Input: part model. Units: mm. Frame: model coordinates. A direction names the side the tool comes from. Coordinates: 2 decimals unless noted, no trailing zeros. Write each loop counter-clockwise with the first axis right and the second up, starting at its lowest first coordinate (ties: lowest second). Pieces come first, ordered by that corner, then holes. Notation, with made-up numbers: M 62,88.25 L 83,88.25 A36 ccw 83,125.25 Z; hole C 10,0.25 d8. An arc over 180 degrees is marked long. Use one line per item in the form item = value.
from build123d import *

# Parameters (mm, degrees)
EXTRUDE003_DEPTH = 5
EXTRUDE002_DEPTH = 5


with BuildPart() as extrude003:
    # Sketch010 (on Face2 of Cut) → Extrude003 (new body)
    with BuildSketch(Plane(origin=(0, 0, 0), x_dir=(1, 0, 0), z_dir=(0, 0, -1))):
        with BuildLine():
            Line((-28.464466, 33.464466), (28.464466, 33.464466))
            ThreePointArc((33.464466, 28.464466), (32, 32), (28.464466, 33.464466))
            Line((33.464466, 28.464466), (33.464466, -28.464466))
            ThreePointArc((28.464466, -33.464466), (32, -32), (33.464466, -28.464466))
            Line((28.464466, -33.464466), (-28.464466, -33.464466))
            ThreePointArc((-33.464466, -28.464466), (-32, -32), (-28.464466, -33.464466))
            Line((-33.464466, -28.464466), (-33.464466, 28.464466))
            ThreePointArc((-28.464466, 33.464466), (-32, 32), (-33.464466, 28.464466))
        make_face()
    extrude(amount=EXTRUDE003_DEPTH)


with BuildPart() as obj1:
    # Sketch009 (on Face2 of Cut) → Extrude002 (new body)
    with BuildSketch(Plane(origin=(0, 0, 0), x_dir=(1, 0, 0), z_dir=(0, 0, -1))):
        with BuildLine():
            ThreePointArc((-31.464466, 36.464466), (-35, 35), (-36.464466, 31.464466))
            Line((-36.464466, -31.464466), (-36.464466, 31.464466))
            ThreePointArc((-36.464466, -31.464466), (-35, -35), (-31.464466, -36.464466))
            Line((31.464466, -36.464466), (-31.464466, -36.464466))
            ThreePointArc((31.464466, -36.464466), (35, -35), (36.464466, -31.464466))
            Line((36.464466, 31.464466), (36.464466, -31.464466))
            ThreePointArc((36.464466, 31.464466), (35, 35), (31.464466, 36.464466))
            Line((-31.464466, 36.464466), (31.464466, 36.464466))
        make_face()
    extrude(amount=EXTRUDE002_DEPTH)

    # Cut001: cut Extrude003
    add(extrude003.part, mode=Mode.SUBTRACT)


solid = obj1.part
(1) Set-up query: faces 5 (the cylindrical face through (32, 32, -2)), 6 (the flat face through (36.464, 0, -2)). Return all of +Z, -Z, +X, -X, +Y, -Y with unobstructed straight access to the full face (end or side cutting, diameter ignored); none if empty.
Computed:
face_5 = +Z, -Z
face_6 = +Z, -Z, +X, +Y, -Y
(2) Pull-direction query (X, two-part tool) for faces 1 (the flat face through (0, 35, 0)), 2 (the cylindrical face through (-35, -35, -2)), 3 (the flat face through (-33.464, 0, -2)), 4 (the cylindrical face through (-32, 32, -2)); classes: pulls with the +X half, pulls with the -X half, needs draft (parallel to the pull), parting line crosses it, or undercut.
Computed:
face_1 = needs draft
face_2 = pulls with the -X half
face_3 = undercut
face_4 = undercut
(3) Section query A-A on y = 10.5. Return the cut outline in (x, z), plus the area to 3 significant figures.
Computed:
outline = M -36.46,-5 L -33.46,-5 L -33.46,0 L -36.46,0 Z; M 33.46,-5 L 36.46,-5 L 36.46,0 L 33.46,0 Z
area = 30.0 mm^2
(4) Line query: probe 1 along Y at (x, z) = (7, -4.6); probe 2 along Y at (x, z) = (30, -2.35). Output: solid intervals per line, ascending.
Computed:
probe_1 = -36.46 to -33.46, 33.46 to 36.46
probe_2 = -36.46 to -33.22, 33.22 to 36.46
(5) Section query C-C on z = -3.3. Return the cut outline in (x, y), plus the area to 3 significant figures.
Computed:
outline = M -36.46,-31.46 A5 ccw -31.46,-36.46 L 31.46,-36.46 A5 ccw 36.46,-31.46 L 36.46,31.46 A5 ccw 31.46,36.46 L -31.46,36.46 A5 ccw -36.46,31.46 Z; hole M -33.46,-28.46 A5 ccw -28.46,-33.46 L 28.46,-33.46 A5 ccw 33.46,-28.46 L 33.46,28.46 A5 ccw 28.46,33.46 L -28.46,33.46 A5 ccw -33.46,28.46 Z
area = 839 mm^2
